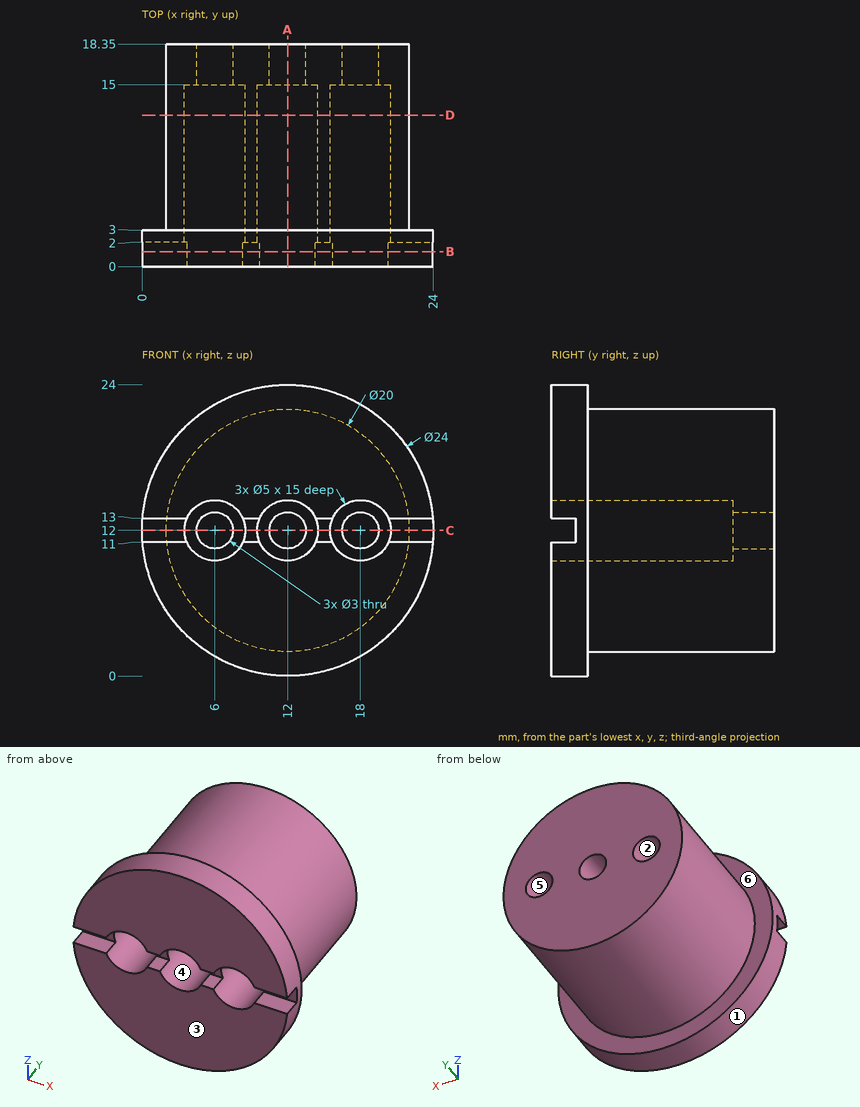
Part print with two shaded views. Sizes in mm from the minimum x, y, z corner. A direction names the side the tool comes from. Coordinates: 2 decimals unless noted, no trailing zeros. Write each loop counter-clockwise with the first axis right and the second up, starting at its lowest first coordinate (ties: lowest second). Pieces come first, ordered by that corner, then holes. Notation, with made-up numbers: (-18, 33.25) - (-8, 33.25) arc R18 ccw to (-8, 42.25) - close; hole circle Ø3 at (-12.5, 83.25). An arc over 180 degrees is marked (long way). Put each result on its own line as item: value.
1. Band-saw the part on C-C (z = 12). Give the number of separate pieces and of enclosed holes in the cut face, then the cut area to 3 significant figures.
Final values:
separate pieces: 4
enclosed holes: 0
area: 106 mm²
2. Band-saw the part on D-D (y = 12.5). Write the cut outline in (x, z), then the cut area to 3 significant figures.
Final values:
outline: circle Ø20 at (12, 12); hole circle Ø5 at (6, 12); hole circle Ø5 at (12, 12); hole circle Ø5 at (18, 12)
area: 255 mm²
3. Flat gauge pins, fed straight in: pin 1 Ø1.6 at (x, y) = (21.5, 1.5) entering from +Z (3 decimals); pin 2 Ø0.6 at (x, y) = (2, 1) entering from -Z; pin 3 Ø4 at (y, z) = (6, 12) entering from -X. Where does each tip first touch, or does it go through?
Final values:
pin 1: stops at z = 20.265
pin 2: stops at z = 4.94
pin 3: stops at x = 2
4. Probe line 1 along Z through (x, y) = (12, 16.25); line 2 along X through (y, z) = (2.75, 14.25); line 3 along X through (y, z) = (2, 14). List the from-to ranges inside material, lowest first. Write a range as [from, to].
Final values:
line 1: z = [2, 10.5], [13.5, 22]
line 2: x = [0.21, 4.91], [7.09, 10.91], [13.09, 16.91], [19.09, 23.79]
line 3: x = [0.17, 4.5], [7.5, 10.5], [13.5, 16.5], [19.5, 23.83]
5. Band-saw the part on A-A (x = 12). Write the cut outline in (y, z).
Final values:
outline: (0, 0) - (3, 0) - (3, 2) - (18.35, 2) - (18.35, 10.5) - (15, 10.5) - (15, 9.5) - (0, 9.5) - close; (0, 14.5) - (15, 14.5) - (15, 13.5) - (18.35, 13.5) - (18.35, 22) - (3, 22) - (3, 24) - (0, 24) - close
6. 3-axis set-ups, long thin cutter, end or side, ignore diameter. For the marked faces 4, 5 and 6: which of +Z, -Z, +X, -X, +Y, -Y reach the whole face in a straight line?
Final values:
face 4: -Y
face 5: +Y, -Y
face 6: +Y
7. Band-saw the part on B-B (y = 1.25). Write the cut outline in (x, z).
Final values:
outline: (0.04, 11) arc R12 ccw to (23.96, 11) - (20.29, 11) arc R2.5 cw to (15.71, 11) - (14.29, 11) arc R2.5 cw to (9.71, 11) - (8.29, 11) arc R2.5 cw to (3.71, 11) - close; (0.04, 13) - (3.71, 13) arc R2.5 cw to (8.29, 13) - (9.71, 13) arc R2.5 cw to (14.29, 13) - (15.71, 13) arc R2.5 cw to (20.29, 13) - (23.96, 13) arc R12 ccw to start
8. Two-plate mould, pull along Z, no slides. Class the marked faces 1, 2 and 3: +Z half, -Z half, draft (parallel to the pull), parting line (faces both ways), or undercut.
Final values:
face 1: parting line
face 2: undercut
face 3: draft
